CAD build for the part. Positions are in the model's coordinates, mm. A direction names the side the tool comes from. Coordinates: 2 decimals unless noted, no trailing zeros. Order: outer loops, then holes, each group sorted by start corner. A loop starts at its lowest first (then second) coordinate and runs counter-clockwise, first axis right, second up. Notation, with made-up numbers: (-33.5, 4) - (-5.5, 4) arc R17 ccw to (-5.5, 22) - close; hole circle Ø4 at (-20.75, 63). An arc over 180 degrees is marked (long way). Use one line per item in the form item = value.
```python
from build123d import *

# Parameters (mm, degrees)
SKETCH001_R       = 1.3
PAD001_DEPTH      = 19.05
PAD001_DEPTH_BACK = 3.5
SKETCH_R          = 25.4
SKETCH_R_2        = 2.225
PAD_DEPTH         = 38.1
FILLET_R          = 0.5


with BuildPart() as pad001:
    # Sketch001 → Pad001 (new body, two sides)
    with BuildSketch(Plane.XY.offset(0.5)) as pad001_sk:
        Circle(SKETCH001_R)
        with Locations((36.32, 0)):
            Circle(SKETCH001_R)
    extrude(amount=PAD001_DEPTH)
    extrude(pad001_sk.sketch, amount=-PAD001_DEPTH_BACK)


with BuildPart() as obj1:
    # Sketch → Pad (new body)
    with BuildSketch(Plane.XY.offset(0.1)):
        with Locations((18.16, 0)):
            Circle(SKETCH_R)
        with Locations((18.16, 0)):
            Circle(SKETCH_R_2, mode=Mode.SUBTRACT)
    extrude(amount=PAD_DEPTH)

    # Fillet
    fillet_edges = [obj1.edges().sort_by_distance(p)[0] for p in [
        (15.935, 0, 38.2),
        (-7.24, 0, 38.2),
        (-7.24, 0, 0.1),
    ]]
    fillet(fillet_edges, radius=FILLET_R)

    # obj1: union Pad001
    add(pad001.part)


solid = obj1.part
```
Item 1: Two-plate mould, pull along Y, no slides. Class faces 1 (the face through (-0.17, 1.29, -1.43)), 2 (the face through (23, 0, 0.1)), 3 (the face through (20.28, 0.67, 18.64)): +Y half, -Y half, draft (parallel to the pull), parting line (faces both ways), or undercut.
Derived:
face_1 = parting line
face_2 = draft
face_3 = undercut
Item 2: Cut at C-C, the plane z = 5.5. Write the cut outline in (x, y) (3 decimals), plus the area to 3 significant figures.
Derived:
outline = circle Ø50.8 at (18.16, 0); hole circle Ø4.45 at (18.16, 0)
area = 2,010 mm²
Item 3: 3-axis set-ups, long thin cutter, end or side, ignore diameter. For faces 4 (the face through (29.881, -22.534, 18.89)), 5 (the face through (37.56, 0.39, -1.43)): which of +Z, -Z, +X, -X, +Y, -Y reach the whole face in a straight line?
Derived:
face_4 = +Z, -Z
face_5 = -Z
Item 4: Cut at B-B, the plane y = 0. Write the cut outline in (x, z) (3 decimals), plus the area to 3 significant figures.
Derived:
outline = (-7.24, 0.6) arc R0.5 ccw to (-6.74, 0.1) - (-1.3, 0.1) - (-1.3, -3) - (1.3, -3) - (1.3, 0.1) - (15.935, 0.1) - (15.935, 37.7) arc R0.5 ccw to (15.435, 38.2) - (-6.74, 38.2) arc R0.5 ccw to (-7.24, 37.7) - close; (20.385, 0.1) - (35.02, 0.1) - (35.02, -3) - (37.62, -3) - (37.62, 0.1) - (43.06, 0.1) arc R0.5 ccw to (43.56, 0.6) - (43.56, 37.7) arc R0.5 ccw to (43.06, 38.2) - (20.885, 38.2) arc R0.5 ccw to (20.385, 37.7) - close
area = 1,780 mm²
Item 5: Drop flat-ended pins along their axis: pin 1 (10 mm diameter, centred on y = 19.5, z = 20, fed in from +X); pin 2 (4 mm diameter, centred on y = -17.5, z = 24, fed in from +X); pin 3 (1.5 mm diameter, centred on x = 3, z = 10, fed in from +Y); pin 4 (3.5 mm diameter, centred on x = 18.16, y = 0, fed in from -Z). Give the stop position or say it passes through.
Derived:
pin_1 = 39.01
pin_2 = 38.28
pin_3 = 20.92
pin_4 = through
Item 6: Drill centre lines: line 1 (Y direction, x = 18, z = 9); line 2 (Z direction, x = 31, y = -15); line 3 (X direction, y = -2, z = 22.5) (3 decimals). Where is each one in solid material? Low to high. Write a range as [from, to].
Derived:
line_1 = [-25.4, -2.22], [2.22, 25.4]
line_2 = [0.1, 38.2]
line_3 = [-7.161, 17.185], [19.135, 43.481]
Item 7: Cut at A-A, the plane x = 18.16. Write the cut outline in (y, z) (3 decimals), plus the area to 3 significant figures.
Derived:
outline = (-25.4, 0.6) arc R0.5 ccw to (-24.9, 0.1) - (-2.225, 0.1) - (-2.225, 37.7) arc R0.5 ccw to (-2.725, 38.2) - (-24.9, 38.2) arc R0.5 ccw to (-25.4, 37.7) - close; (2.225, 0.1) - (24.9, 0.1) arc R0.5 ccw to (25.4, 0.6) - (25.4, 37.7) arc R0.5 ccw to (24.9, 38.2) - (2.725, 38.2) arc R0.5 ccw to (2.225, 37.7) - close
area = 1,770 mm²
